Drawing for the job (mm, zero at the part's lowest x, y, z). A direction names the side the tool comes from. Round coordinates to 2 decimals unless told otherwise and drop trailing zeros. Write each loop counter-clockwise with the first axis right and the second up, starting at its lowest first coordinate (ties: lowest second). Pieces come first, ordered by that corner, then holes.
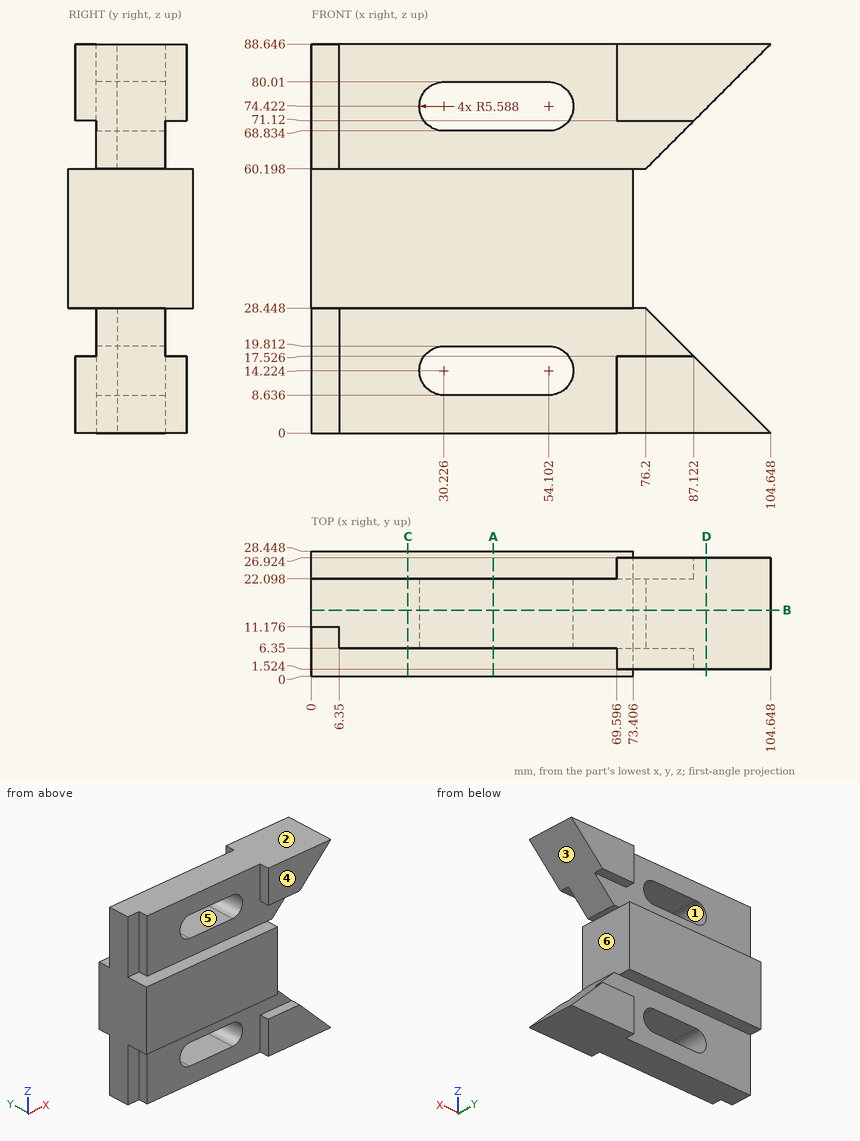
Q1. Saw through at C-C, the plane x = 22. Write the cut outline in (y, z), and give its area (3 significant figures).
Q2. Tool access for the marked faces 4, 5 and 6: list every direction of +Z, -Z, +X, -X, +Y, -Y with a clear straight run to the whole face (end or side of a thin tool).
Q3. Two-plate mould, pull along X, no slides. Class the marked faces 1, 2 and 3: released by +X, released by -X, zero draft, split by the parting line, or undercut.
Q4. Saw through at A-A, the plane x = 41.5. Write the cut outline in (y, z), and give its area (3 significant figures).
Q5. Saw through at D-D, the plane x = 90. Write the cut outline in (y, z), and give its area (3 significant figures).
Q6. Wall check: line 1 (Z direction, x = 70, y = 26); line 2 (Z direction, x = 38, y = 16); line 3 (Y direction, x = 18.5, z = 64). Give the ranges that are in metal, low to high.
Q7. Saw through at B-B, the plane y = 15. Write the cut outline in (x, z).
Q8. Drop flat-ended pins along their axis: P1, Ø8, axis at x = 14.5, z = 21, coming from the -Y side; P2, Ø5, axis at y = 5.5, z = 17.5, coming from the -X side; P3, Ø8.5, axis at x = 41, z = 70, coming from the +Y side. Give the stop position or say it passes through.
Computed:
1. outline: (0, 28.45) - (6.35, 28.45) - (6.35, 0) - (22.1, 0) - (22.1, 28.45) - (28.45, 28.45) - (28.45, 60.2) - (22.1, 60.2) - (22.1, 88.65) - (6.35, 88.65) - (6.35, 60.2) - (0, 60.2) - close
1. area: 1,800 mm2
2. face 4: +Z, +X, -X, -Y
2. face 5: +Y, -Y
2. face 6: +X, +Y, -Y
3. face 1: undercut
3. face 2: zero draft
3. face 3: released by +X
4. outline: (0, 28.45) - (6.35, 28.45) - (6.35, 19.81) - (22.1, 19.81) - (22.1, 28.45) - (28.45, 28.45) - (28.45, 60.2) - (22.1, 60.2) - (22.1, 68.83) - (6.35, 68.83) - (6.35, 60.2) - (0, 60.2) - close; (6.35, 0) - (22.1, 0) - (22.1, 8.64) - (6.35, 8.64) - close; (6.35, 80.01) - (22.1, 80.01) - (22.1, 88.65) - (6.35, 88.65) - close
4. area: 1,450 mm2
5. outline: (1.52, 0) - (26.92, 0) - (26.92, 14.65) - (1.52, 14.65) - close; (1.52, 74) - (26.92, 74) - (26.92, 88.65) - (1.52, 88.65) - close
5. area: 744 mm2
6. line 1: z = 0 to 17.53, 28.45 to 60.2, 71.12 to 88.65
6. line 2: z = 0 to 8.64, 19.81 to 68.83, 80.01 to 88.65
6. line 3: y = 6.35 to 22.1
7. outline: (0, 0) - (104.65, 0) - (76.2, 28.45) - (73.41, 28.45) - (73.41, 60.2) - (76.2, 60.2) - (104.65, 88.65) - (0, 88.65) - close; hole (30.23, 8.64) - (54.1, 8.64) arc R5.59 ccw to (54.1, 19.81) - (30.23, 19.81) arc R5.59 ccw to start; hole (30.23, 68.83) - (54.1, 68.83) arc R5.59 ccw to (54.1, 80.01) - (30.23, 80.01) arc R5.59 ccw to start
8. P1: stops at y = 6.35
8. P2: stops at x = 6.35
8. P3: stops at y = 22.1
